The listing builds one solid part. Answer for the finished solid, in the listing's coordinates (mm). Round coordinates to 2 decimals unless told otherwise and drop trailing zeros. Write each loop counter-clockwise with the first axis right and the second up, starting at its lowest first coordinate (ties: lowest second). Pieces come first, ordered by that corner, then holes. Notation, with made-up numbers: (-13, 45.25) - (-3, 45.25) arc R6 ccw to (-3, 51.25) - close; hole circle Ø3 at (-10.5, -11.5). An arc over 180 degrees is marked (long way). Use a Markdown table: item, result. Add a question column.
1) Each of these flat-tipped pins is pushed along its axis until it touches: P1, Ø1, axis at y = 78.5, z = 2, coming from the -X side; P2, Ø6, axis at y = 51, z = 4, coming from the +X side; P3, Ø3, axis at x = 75.5, z = 5, coming from the +Y side. Where does it stop, or does it pass through?
2) Find the intervals of material crossed by probe 1 along X at (y, z) = (61, 7.75); probe 2 along X at (y, z) = (102.5, 5.25); probe 3 along X at (y, z) = (97, 5.25), in increasing order. Write a range as from..to.
3) A cutting plane is placed at A-A (y = 68). Give the vertices of the cut face in (x, z).
4) A cutting plane is placed at B-B (z = 2.5). Give the vertices of the cut face in (x, y), then the cut area to 3 significant figures.
5) A cutting plane is placed at C-C (x = -62.5). Give the vertices of the cut face in (y, z), then the cut area to 3 significant figures.
6) Determine the mould class of faces 1 (the flat face through (1, 34, 0)), 2 (the cylindrical face through (14.78, 86.1, 4.93)), 3 (the flat face through (-70.1, 60.09, 4.93)) for opening direction Y: +Y half, -Y half, draft (parallel to the pull), parting line (faces both ways), or undercut.
```python
from build123d import *

# Parameters (mm, degrees)
SKETCH_R  = 27.5
PAD_DEPTH = 10


with BuildPart() as part:
    # Sketch → Pad (new body)
    with BuildSketch(Plane.XY):
        with BuildLine():
            Line((-95, 0), (-95, 25.815306))
            Line((-95, 25.815306), (-44.495935, 95.328189))
            ThreePointArc((0, 118), (-24.969477, 112.005359), (-44.495935, 95.328189))
            ThreePointArc((44.495935, 95.328189), (24.969477, 112.005359), (0, 118))
            Line((95, 25.815306), (44.495935, 95.328189))
            Line((95, 0), (95, 25.815306))
            Line((-95, 0), (95, 0))
        make_face()
        with Locations((0, 62.91)):
            Circle(SKETCH_R, mode=Mode.SUBTRACT)
    extrude(amount=PAD_DEPTH)


solid = part.part
```
Entries:
| question | item | result |
|---|---|---|
| 1 | P1 | stops at x = -57.09 |
| 1 | P2 | stops at x = 78.88 |
| 1 | P3 | stops at y = 54.72 |
| 2 | probe 1 | x = -69.44..-27.43, 27.43..69.44 |
| 2 | probe 2 | x = -38.27..38.27 |
| 2 | probe 3 | x = -43.23..43.23 |
| 3 | outline | (-64.35, 0) - (-27.02, 0) - (-27.02, 10) - (-64.35, 10) - close; (27.02, 0) - (64.35, 0) - (64.35, 10) - (27.02, 10) - close |
| 4 | outline | (-95, 0) - (95, 0) - (95, 25.82) - (44.5, 95.33) arc R55 ccw to (0, 118) arc R55 ccw to (-44.5, 95.33) - (-95, 25.82) - close; hole circle Ø55 at (0, 62.91) |
| 4 | area | 13,600 mm² |
| 5 | outline | (0, 0) - (70.55, 0) - (70.55, 10) - (0, 10) - close |
| 5 | area | 705 mm² |
| 6 | face 1 | draft |
| 6 | face 2 | undercut |
| 6 | face 3 | +Y half |
